Source: CAD feature listing. Evaluate the final solid. Frame: model axes, mm. A direction names the side the tool comes from. Round coordinates to 2 decimals unless told otherwise and drop trailing zeros. Order: outer loops, then holes, each group sorted by start corner. A loop starts at its lowest first (then second) coordinate and runs counter-clockwise, first axis right, second up. Notation, with made-up numbers: M -31.75,18.5 L -5.75,18.5 A30 cw -5.75,43.5 Z; hole C -19,49 d6. An arc over 180 degrees is marked long. Use one line per item in the form item = value. Start each with the question number.
Q1. Section B-B (y = -65). Give the number of separate pieces and of enclosed holes in the cut face, plus the area to 3 significant figures.
Q2. Pull-direction query (Y, two-part tool) for faces 4 (the cylindrical face through (63.799, -67.918, 9.138)), 5 (the flat face through (63.28, -62.82, 8.02)), 6 (the cylindrical face through (-5.866, 1.261, 7.888)), 7 (the flat face through (32.42, 3.13, 7.89)); classes: pulls with the +Y half, pulls with the -Y half, needs draft (parallel to the pull), parting line crosses it, or undercut.
Q3. Reachability of faces 1 (the flat face through (50.472, -20.54, 8.112)), 2 (the flat face through (13.525, 3.524, 7.888)), 3 (the cylindrical face through (97.624, -70.942, 8.059)) from +Z, -Z, +X, -X, +Y, -Y: full face, straight path, thin tool, end or side. Return the list, or none.
Q4. Section C-C (y = -35.5). Return the cut outline in (x, z).
Q5. Material intervals for probe 1 along X at (y, z) = (-16, 8); probe 2 along Y at (x, z) = (0, 12.75); probe 3 along Y at (x, z) = (-0.5, 9), sorted ascending.
Q6. Contact query for flat-ended pins moving along their axis: pin 1 (1.8 mm diameter, centred on x = 0, y = 0, fed in from +Z); pin 2 (2 mm diameter, centred on y = -57.5, z = 1.5, fed in from +X); pin 3 (8 mm diameter, centred on x = 100, z = 14, fed in from +Y); pin 4 (8 mm diameter, centred on y = -33, z = 11.5, fed in from -X). Output: stop coordinate, or through.
Q7. Section A-A (x = 38.5). Return the cut outline in (y, z).
from build123d import *

# Parameters (mm, degrees)
SKETCH_1_R          = 1.5
EXTRUDE_1_DEPTH     = 16
SKETCH_2_R          = 1.35
CUT_EXTRUDE_1_DEPTH = 10
CUT_EXTRUDE_2_DEPTH = 33
EXTRUDE_3_DEPTH     = 16
SKETCH_6_R          = 1.5
CUT_EXTRUDE_3_DEPTH = 48
EXTRUDE_4_DEPTH     = 16


with BuildPart() as part:
    # 草图1 → 凸台-拉伸1 (new body)
    with BuildSketch(Plane.XY):
        with BuildLine():
            Line((1.126380295, 5.893323971), (37.220974686, -1.005370225))
            Line((37.220974686, -1.005370225), (63.227984205, -49.979924472))
            Line((63.227984205, -49.979924472), (112.538061605, -75))
            Line((112.538061605, -75), (53.330616959, -72.391905084))
            Line((53.330616959, -72.391905084), (49.915441771, -64.88738307))
            Line((49.915441771, -64.88738307), (26.682733599, -13.835720919))
            Line((26.682733599, -13.835720919), (-1.643050648, -5.77064854))
            ThreePointArc((-1.643050648, -5.77064854), (-5.837705093, 1.386073321), (1.126380295, 5.893323971))
        make_face()
        Circle(SKETCH_1_R, mode=Mode.SUBTRACT)
    extrude(amount=EXTRUDE_1_DEPTH)

    # 草图2 → 切除-拉伸1 (cut)
    with BuildSketch(Plane(origin=(-3.079413203, -69.907036606, 0), x_dir=(0.9990312032291818, -0.044007442262116094, 0), z_dir=(-0.044007442262116094, -0.9990312032291818, 0))):
        with Locations((66, 8)):
            Circle(SKETCH_2_R)
        with Locations((102, 8)):
            Circle(SKETCH_2_R)
        with Locations((84, 8)):
            Circle(SKETCH_2_R)
    extrude(amount=-CUT_EXTRUDE_1_DEPTH, mode=Mode.SUBTRACT)

    # 草图3 → 切除-拉伸2 (cut)
    with BuildSketch(Plane.XY.offset(16)):
        Polygon((26.682733599, -13.835720919), (54.911117554, -72.461526322), (53.330616959, -72.391905084), align=None)
    extrude(amount=-CUT_EXTRUDE_2_DEPTH, mode=Mode.SUBTRACT)

    # 草图5 → 凸台-拉伸3 (add)
    with BuildSketch(Plane(origin=(0, 0, 0), x_dir=(-1, 0, 0), z_dir=(0, 0, -1))):
        Polygon((-37.220974686, -1.005370225), (-27.480137518, 7.389214918), (-26.275532527, 1.086612233), align=None)
    extrude(amount=-EXTRUDE_3_DEPTH)

    # 草图6 → 切除-拉伸3 (cut)
    with BuildSketch(Plane(origin=(0, 0, 0), x_dir=(-1, 0, 0), z_dir=(0, 0, -1))):
        with Locations((-47.911117554, -40.461526322)):
            Circle(SKETCH_6_R)
    extrude(amount=-CUT_EXTRUDE_3_DEPTH, mode=Mode.SUBTRACT)

    # 草图7 → 凸台-拉伸4 (add)
    with BuildSketch(Plane.XY.offset(16)):
        Polygon((46.698574744, -18.852913898), (50.712719625, -15.723743191), (50.224479445, -25.492647349), align=None)
    extrude(amount=-EXTRUDE_4_DEPTH)


solid = part.part
Results list:
q1.separate_pieces = 1
q1.enclosed_holes = 2
q1.area = 653 mm2
q2.face_4 = undercut
q2.face_5 = undercut
q2.face_6 = parting line crosses it
q2.face_7 = pulls with the +Y half
q3.face_1 = +Z, -Z, +X
q3.face_2 = +Z, -Z, +Y
q3.face_3 = none
q4.outline = M 37.11,0 L 55.54,0 L 55.54,16 L 37.11,16 Z
q5.probe_1 = 27.72 to 45.18, 50.36 to 50.7
q5.probe_2 = -6.24 to -1.5, 1.5 to 6
q5.probe_3 = -6.1 to -1.41, 1.41 to 5.98
q6.pin_1 = through
q6.pin_2 = 80.02
q6.pin_3 = -66.61
q6.pin_4 = 33.98
q7.outline = M -38.38,0 L -3.41,0 L -3.41,16 L -38.38,16 Z
